Drawing for the job (mm, zero at the part's lowest x, y, z). A direction names the side the tool comes from. Round coordinates to 2 decimals unless told otherwise and drop trailing zeros. Order: outer loops, then holes, each group sorted by start corner. A loop starts at its lowest first (then second) coordinate and runs counter-clockwise, first axis right, second up. Notation, with made-up numbers: M 0,46 L 17,46 A21 ccw 17,62 Z; hole C -38.5,68 d4. An arc over 180 degrees is marked long. Answer as CSV lines item,"result". Start each with the question number.
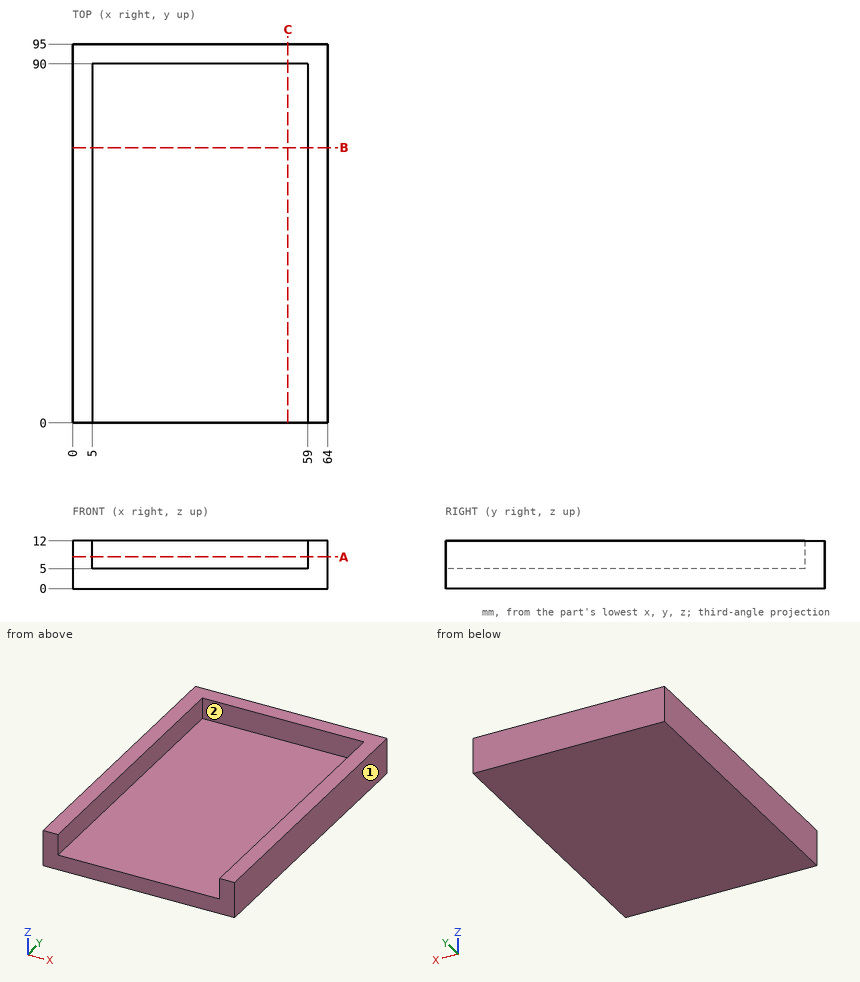
Q1. Drop flat-ended pins along their axis: P1, Ø1.5, axis at x = 14.5, y = 10, coming from the -Z side; P2, Ø2, axis at x = 27.5, z = 7.5, coming from the -Y side; P3, Ø2, axis at x = 8.5, y = 45.5, coming from the +Z side. Give the stop position or say it passes through.
Q2. Probe line 1 along X through (y, z) = (11, 9.5); line 2 along Y through (x, z) = (41.5, 10); line 3 along Z through (x, y) = (43, 39). List the from-to ranges inside material, lowest first. Write a range as from..to.
Q3. Band-saw the part on C-C, the plane x = 54. Write the cut outline in (y, z), then the cut area to 3 significant figures.
Q4. Tool access for the marked faces 1 and 2: list every direction of +Z, -Z, +X, -X, +Y, -Y with a clear straight run to the whole face (end or side of a thin tool).
Q5. Band-saw the part on A-A, the plane z = 8. Write the cut outline in (x, y).
Q6. Band-saw the part on B-B, the plane y = 69. Write the cut outline in (x, z), then the cut area to 3 significant figures.
Answer:
1,P1,"stops at z = 0"
1,P2,"stops at y = 90"
1,P3,"stops at z = 5"
2,line 1,"x = 0..5, 59..64"
2,line 2,"y = 90..95"
2,line 3,"z = 0..5"
3,outline,"M 0,0 L 95,0 L 95,12 L 90,12 L 90,5 L 0,5 Z"
3,area,"510 mm^2"
4,face 1,"+Z, -Z, +X, +Y, -Y"
4,face 2,"+Z, -Y"
5,outline,"M 0,0 L 5,0 L 5,90 L 59,90 L 59,0 L 64,0 L 64,95 L 0,95 Z"
6,outline,"M 0,0 L 64,0 L 64,12 L 59,12 L 59,5 L 5,5 L 5,12 L 0,12 Z"
6,area,"390 mm^2"
